Read the model definition and answer for the solid it produces. Units are mm, in the model's axes. A direction names the side the tool comes from. Round coordinates to 2 decimals unless told otherwise and drop trailing zeros. Order: outer loops, then holes, each group sorted by start corner. A loop starts at its lowest first (then second) coordinate and runs counter-clockwise, first axis right, second up. Notation, with made-up numbers: (80, -14.75) -> (95, -14.75) arc R10 ccw to (95, -3.75) -> close; hole circle Ø6 at (-33.75, 3). An arc over 180 degrees is marked (long way). Answer as a JSON object with one key per item and string values. Group by question number.
Item 1: Consider probe 1 along Y at (x, z) = (33, -9); probe 2 along X at (y, z) = (31.5, 5); probe 3 along X at (y, z) = (32.5, -3). Determine where each line is inside the solid, lowest interval first. Write a range as from..to.
Item 2: For faces 4 (the cylindrical face through (37.794, 8.026, -28.979)), 5 (the flat face through (-20, 1.588, 1)), determine the directions among +Z, -Z, +X, -X, +Y, -Y from which every point of the face is accessible in a straight line to the end or side of a thin tool.
Item 3: Section D-D, the plane y = 21 is taken. Write down the section's boundary in (x, z), plus the area to 3 significant figures.
Item 4: Section C-C, the plane z = 26.5 is taken. Write down the section's boundary in (x, y).
Item 5: The mould has two halves that part along Z. Classify faces 1 (the cylindrical face through (-16.72, 0.8, 5.26)), 2 (the flat face through (-20, 14.288, 1)), 3 (the cylindrical face through (-25.26, 7.85, -31.34)): pulls with the +Z half, pulls with the -Z half, needs draft (parallel to the pull), parting line crosses it, or undercut.
Item 6: Given P1, Ø18.5, axis at x = 23.53, z = -23.53, coming from the +Y side; P2, Ø5, axis at x = 32.5, z = 38, coming from the -Y side; P3, Ø3, axis at x = -8.5, y = 46.5, coming from the +Z side, each flat-ended and moving along its own axis, determine where each tip first touches the part or whether it passes through.
Autodesk Inventor part; units mm, degrees
ref_plane "YZ Plane" through (0, 0, 0) normal (1, 0, 0) x (0, 1, 0)
ref_plane "XZ Plane" through (0, 0, 0) normal (0, 1, 0) x (-1, 0, 0)
ref_plane "XY Plane" through (0, 0, 0) normal (0, 0, 1) x (1, 0, 0)
sketch "Sketch1" plane through (0, 0, 0) normal (0, 0, 1) x (1, 0, 0)
  line L0 (0, 0) -> (0, 52.3875) construction
  line L1 (-7.874, 52.3875) -> (-7.874, 0)
  line L2 (-7.874, 0) -> (-17.526, 0)
  line L3 (-17.526, 0) -> (-17.526, 1.5875)
  line L4 (-17.526, 1.5875) -> (-47.625, 1.5875)
  line L5 (-47.625, 1.5875) -> (-47.625, 14.2875)
  line L6 (-47.625, 14.2875) -> (-19.05, 14.2875)
  line L7 (-19.05, 14.2875) -> (-10.668, 50.7744)
  line L8 (-10.668, 50.7744) -> (-7.874, 52.3875)
  line L9 (-33.274, 14.2875) -> (-33.274, 1.5875) construction
  dimension "WB" = 15.748
  dimension "d1" = 1.5875
  dimension "WL" = 50.8
  dimension "Thickness" = 12.7
  dimension "R" = 35.052
  dimension "OD" = 95.25
  dimension "HB" = 38.1
  dimension "HT" = 21.336
  dimension "d8" = 60
  dimension "BC" = 66.548
revolve "Revolution1" add sketch "Sketch1" angle 360 about axis through (0, 0, 0) along (0, 1, 0)
sketch "Sketch2" plane through (0, 14.2875, 0) normal (0, 1, 0) x (1, 0, 0)
  line L0 (0, 0) -> (0, 47.625) construction
  circle A0 centre (0, 0) radius 47.625
  line L1 (0, 0) -> (23.5283, 23.5283) construction
  dimension "d11" = 45
  dimension "d12" = 33.274
hole "Hole1" at (23.5283, 14.2875, -23.5283) direction (0, -1, 0) diameter 16.002 depth 12.7
pattern_circular "Circular Pattern1" count 4 over 360 about axis through (0, -10, 0) along (0, 1, 0) of "Hole1"
equation "\"d12\" = 0.5 * BC"
properties part number "ANSI-B300-0.5W"
Values found:
{
 "1": {"probe 1": "1.59..14.29", "probe 2": "-14.24..-6.08, 6.08..14.24", "probe 3": "-14.56..-7.28, 7.28..14.56"},
 "2": {"face 4": "+Y, -Y", "face 5": "-Y"},
 "3": {"outline": "circle Ø35.02 at (0, 0); hole circle Ø15.75 at (0, 0)", "area": "768 mm2"},
 "4": {"outline": "(-39.57, 1.59) -> (-30.96, 1.59) -> (-30.96, 14.29) -> (-39.57, 14.29) -> close; (-16.1, 1.59) -> (16.1, 1.59) -> (16.1, 14.29) -> (-16.1, 14.29) -> close; (30.96, 1.59) -> (39.57, 1.59) -> (39.57, 14.29) -> (30.96, 14.29) -> close"},
 "5": {"face 1": "parting line crosses it", "face 2": "needs draft", "face 3": "undercut"},
 "6": {"P1": "y = 14.29", "P2": "y = 1.59", "P3": "z = 9.39"}
}
